from build123d import *

# Parameters (mm, degrees)
SKETCH1_W           = 69
SKETCH1_H           = 54
BOSS_EXTRUDE1_DEPTH = 2
SKETCH2_R           = 2.1
SKETCH2_R_2         = 1.6
BOSS_EXTRUDE2_DEPTH = 5


with BuildPart() as part:
    # Sketch1 → Boss-Extrude1 (new body)
    with BuildSketch(Plane(origin=(0, 0, 0), x_dir=(1, 0, 0), z_dir=(0, 1, 0))):
        Rectangle(SKETCH1_W, SKETCH1_H)
    extrude(amount=BOSS_EXTRUDE1_DEPTH)

    # Sketch2 → Boss-Extrude2 (add)
    # profile 1 of 4: a face of its own
    with BuildSketch(Plane(origin=(0, 2, 0), x_dir=(1, 0, 0), z_dir=(0, 1, 0))):
        with Locations(Location((-19.4, 23.55, 0), (0, 0, 90))):
            Circle(SKETCH2_R)
        with Locations(Location((-19.4, 23.55, 0), (0, 0, 270))):
            Circle(SKETCH2_R_2, mode=Mode.SUBTRACT)
    # profile 2 of 4: a face of its own
    with BuildSketch(Plane(origin=(0, 2, 0), x_dir=(1, 0, 0), z_dir=(0, 1, 0))):
        with Locations(Location((31.4, 8.35, 0), (0, 0, 90))):
            Circle(SKETCH2_R)
        with Locations(Location((31.4, 8.35, 0), (0, 0, 270))):
            Circle(SKETCH2_R_2, mode=Mode.SUBTRACT)
    # profile 3 of 4: a face of its own
    with BuildSketch(Plane(origin=(0, 2, 0), x_dir=(1, 0, 0), z_dir=(0, 1, 0))):
        with Locations(Location((31.4, -19.55, 0), (0, 0, 90))):
            Circle(SKETCH2_R)
        with Locations(Location((31.4, -19.55, 0), (0, 0, 270))):
            Circle(SKETCH2_R_2, mode=Mode.SUBTRACT)
    # profile 4 of 4: a face of its own
    with BuildSketch(Plane(origin=(0, 2, 0), x_dir=(1, 0, 0), z_dir=(0, 1, 0))):
        with Locations(Location((-20.5, -24.25, 0), (0, 0, 90))):
            Circle(SKETCH2_R)
        with Locations(Location((-20.5, -24.25, 0), (0, 0, 270))):
            Circle(SKETCH2_R_2, mode=Mode.SUBTRACT)
    extrude(amount=BOSS_EXTRUDE2_DEPTH)


solid = part.part
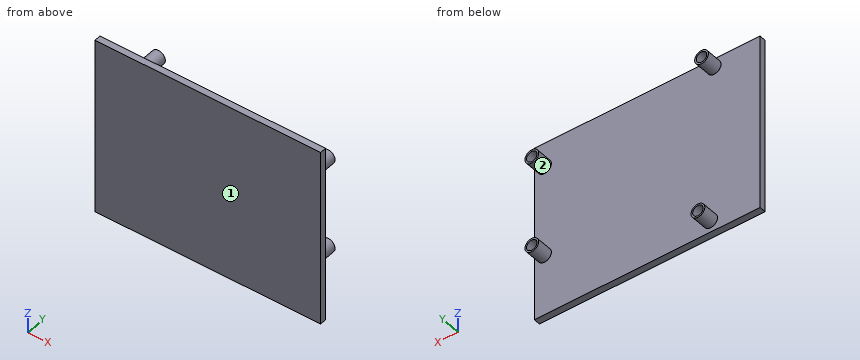
Verification items for the finished model (mm, model axes). Face numbers are marked on the shaded views. Round coordinates to 2 decimals unless told otherwise and drop trailing zeros. Loops run counter-clockwise (first coordinate to the right, second up) from the corner with the lowest first, then second, coordinate; pieces in that order, holes last. Notation, with made-up numbers: (15.5, -33.5) - (50.5, -33.5) arc R16 cw to (50.5, -21.5) - close; hole circle Ø11 at (36, -7). An arc over 180 degrees is marked (long way). Use a Markdown table: item, result. Add a question column.
1. Thickness scan on probe 1 along X at (y, z) = (5.7, -8.35); probe 2 along X at (y, z) = (5.25, 24.25); probe 3 along Y at (x, z) = (23, 22). Record the ranges inside material, lowest first. Write a range as [from, to].
2. Section check B-B, the plane z = 19.55. Record the boundary of the cut face in (x, y), plus the area to 3 significant figures.
3. Section check A-A, the plane y = 5.5. Record the boundary of the cut face in (x, z).
4. Section check D-D, the plane x = 24. Record the boundary of the cut face in (y, z).
5. Release check for a two-part mould opening along Z. For the marked faces 1 and 2 record: released by +Z, released by -Z, zero draft, split by the parting line, or undercut.
6. Section check C-C, the plane x = 31.4. Record the boundary of the cut face in (y, z), plus the area to 3 significant figures.
7. Gauge pin test, flat end, axial feed: pin 1 (1 mm diameter, centred on x = 31.5, z = -8.5, fed in from +Y). Record the tip position at first contact, or that the pin passes through.
Checks:
| question | item | result |
|---|---|---|
| 1 | probe 1 | x = [29.3, 29.8], [33, 33.5] |
| 1 | probe 2 | x = [-22.6, -22.1], [-18.9, -18.4] |
| 1 | probe 3 | y = [0, 2] |
| 2 | outline | (-34.5, 0) - (34.5, 0) - (34.5, 2) - (33.5, 2) - (33.5, 7) - (33, 7) - (33, 2) - (29.8, 2) - (29.8, 7) - (29.3, 7) - (29.3, 2) - (-34.5, 2) - close |
| 2 | area | 143 mm^2 |
| 3 | outline | circle Ø4.2 at (-20.5, 24.25); circle Ø4.2 at (-19.4, -23.55); circle Ø4.2 at (31.4, -8.35); circle Ø4.2 at (31.4, 19.55); hole circle Ø3.2 at (-20.5, 24.25); hole circle Ø3.2 at (-19.4, -23.55); hole circle Ø3.2 at (31.4, -8.35); hole circle Ø3.2 at (31.4, 19.55) |
| 4 | outline | (0, -27) - (2, -27) - (2, 27) - (0, 27) - close |
| 5 | face 1 | zero draft |
| 5 | face 2 | undercut |
| 6 | outline | (0, -27) - (2, -27) - (2, -10.45) - (7, -10.45) - (7, -9.95) - (2, -9.95) - (2, -6.75) - (7, -6.75) - (7, -6.25) - (2, -6.25) - (2, 17.45) - (7, 17.45) - (7, 17.95) - (2, 17.95) - (2, 21.15) - (7, 21.15) - (7, 21.65) - (2, 21.65) - (2, 27) - (0, 27) - close |
| 6 | area | 118 mm^2 |
| 7 | pin 1 | stops at y = 2 |
